Drawing for the job (mm, zero at the part's lowest x, y, z). A direction names the side the tool comes from. Coordinates: 2 decimals unless noted, no trailing zeros. Loops run counter-clockwise (first coordinate to the right, second up) from the corner with the lowest first, then second, coordinate; pieces in that order, holes last. Notation, with made-up numbers: (-23.75, -31.5) -> (32.25, -31.5) arc R26 cw to (32.25, -9.5) -> close; hole circle Ø2 at (-13, 32.5). An arc over 180 degrees is marked (long way). Write item = value, one per line. Start each with the question number.
(1) Band-saw the part on B-B (y = 20). Write the cut outline in (x, z).
(2) Band-saw the part on C-C (z = 52.5). Write the cut outline in (x, y).
(3) Band-saw the part on A-A (x = 25.4). Write the cut outline in (y, z), and give its area (3 significant figures).
(4) Drill centre lines: line 1 (Z direction, x = 25.4, y = 19); line 2 (X direction, y = 20, z = 50) (1 decimal); line 3 (Z direction, x = 119, y = 25). Where is each one in solid material? Low to high. Write a range as from..to.
(5) Band-saw the part on D-D (x = 69.5). Write the cut outline in (y, z), and give its area (3 significant figures).
(6) Tool access for the marked faces 1 and 2: list every direction of +Z, -Z, +X, -X, +Y, -Y with a clear straight run to the whole face (end or side of a thin tool).
(7) Pull direction X, two halves, no side cores. Call the marked faces 3, 4 and 5: +X half, -X half, draft (parallel to the pull), parting line (faces both ways), or undercut.
(8) Flat gauge pins, fed straight in: P1, Ø12, axis at y = 14, z = 48.5, coming from the +X side; P2, Ø6, axis at x = 111.5, y = 13, coming from the +Z side; P3, Ø8, axis at y = 11.5, z = 60.5, coming from the +X side. Where does each tip first touch, or does it go through?
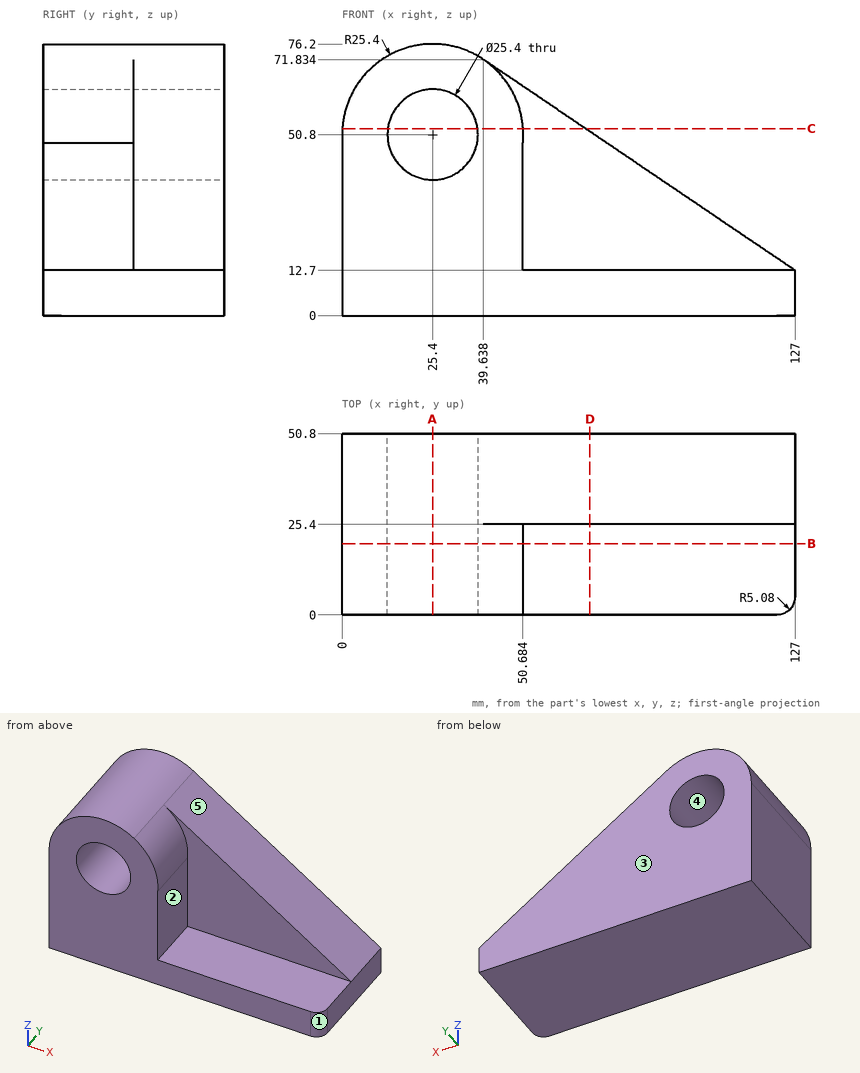
Findings below:
q1.outline = (0, 0) -> (127, 0) -> (127, 12.7) -> (50.68, 12.7) -> (50.68, 48.38) arc R25.4 ccw to (39.64, 71.83) arc R25.4 ccw to (0, 50.8) -> close; hole circle Ø25.4 at (25.4, 50.8)
q2.outline = (0.06, 0) -> (12.81, 0) -> (12.81, 50.8) -> (0.06, 50.8) -> close; (37.99, 0) -> (50.74, 0) -> (50.74, 25.4) -> (68.2, 25.4) -> (68.2, 50.8) -> (37.99, 50.8) -> close
q3.outline = (0, 0) -> (50.8, 0) -> (50.8, 38.1) -> (0, 38.1) -> close; (0, 63.5) -> (50.8, 63.5) -> (50.8, 76.2) -> (0, 76.2) -> close
q3.area = 2,580 mm²
q4.line_1 = 0..38.1, 63.5..76.2
q4.line_2 = 0..12.7, 38.1..50.8
q4.line_3 = 0..12.7
q5.outline = (0, 0) -> (50.8, 0) -> (50.8, 51.62) -> (25.4, 51.62) -> (25.4, 12.7) -> (0, 12.7) -> close
q5.area = 1,630 mm²
q6.face_1 = +Z, -Z, +X, -Y
q6.face_2 = +X, -Y
q7.face_3 = draft
q7.face_4 = undercut
q7.face_5 = +X half
q8.P1 = 50.8
q8.P2 = 12.7
q8.P3 = 50.15
